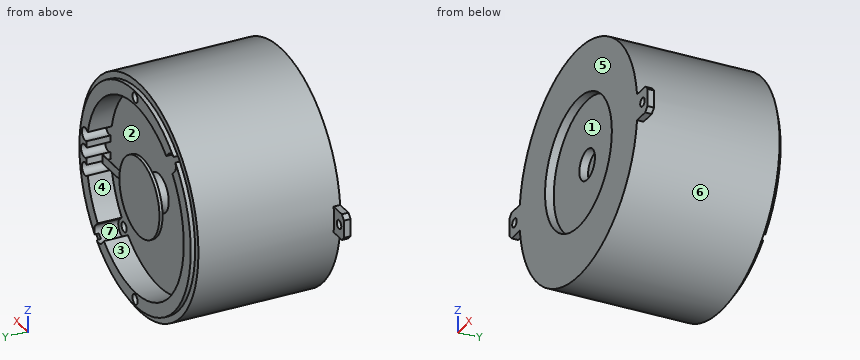
```python
from build123d import *

# Parameters (mm, degrees)
SKETCH_2_R              = 1
EXTRUDE_1_DEPTH         = 1.5
SKETCH_4_R              = 3.5
CUT_EXTRUDE_1_DEPTH     = 2
HOLE_WIZARD_M2_21_D     = 2.3
HOLE_WIZARD_M2_21_DEPTH = 10
HOLE_WIZARD_M2_21_TIP   = 0.690989712
HOLE_WIZARD_M2_22_D     = 2.3
HOLE_WIZARD_M2_22_DEPTH = 10
HOLE_WIZARD_M2_22_TIP   = 0.690989712
SKETCH_18_R             = 2
CUT_EXTRUDE_3_DEPTH     = 5.5
HOLE_WIZARD_M2_23_D     = 2.3
HOLE_WIZARD_M2_23_DEPTH = 15
HOLE_WIZARD_M2_23_TIP   = 0.690989712
CUT_EXTRUDE_START       = -5.5
SKETCH_20_R             = 1.5
CUT_EXTRUDE_4_DEPTH     = 5.5
SKETCH_8_W              = 2
SKETCH_8_H              = 0.05
EXTRUDE_3_DEPTH         = 18
SKETCH_9_R              = 2
CUT_EXTRUDE_2_DEPTH     = 5.5


# Read off the part's stored shape, not the designer's step: Повернуть1
with BuildPart() as part:
    # Повернуть1 outline → Повернуть1 (revolve)
    with BuildSketch(Plane.XY):
        Polygon((0, 26.1), (0, 0), (15, 0), (15, -2), (26.5, -2), (26.5, 30.6), (25, 30.6), (25, 31.6), (21.858230866, 31.6), (21.858230866, 26.1), align=None)
    revolve(axis=Axis((0, 0, 0), (0, 1, 0)))

    # Эскиз2 → Бобышка-Вытянуть1 (add)
    # profile 1 of 2: a face of its own
    with BuildSketch(Plane.XZ.offset(2)):
        Polygon((-31, -2), (-31, 2), (-30, 3), (-26.329641091, 3), (-26.329641091, -3), (-30, -3), align=None)
        with Locations(Location((-28.75, 0, 0), (0, 0, 270))):
            Circle(SKETCH_2_R, mode=Mode.SUBTRACT)
    # profile 2 of 2: a face of its own
    with BuildSketch(Plane.XZ.offset(2)):
        Polygon((30, 3), (26.329641091, 3), (26.329641091, -3), (30, -3), (31, -2), (31, 2), align=None)
        with Locations(Location((28.75, 0, 0), (0, 0, 90))):
            Circle(SKETCH_2_R, mode=Mode.SUBTRACT)
    extrude(amount=-EXTRUDE_1_DEPTH)

    # Эскиз4 → Вырез-Вытянуть1 (cut)
    with BuildSketch(Plane.XZ):
        with Locations(Location((0, 0, 0), (0, 0, 270))):
            Circle(SKETCH_4_R)
    extrude(amount=-CUT_EXTRUDE_1_DEPTH, mode=Mode.SUBTRACT)

    # Эскиз7 → Повернуть2 (revolve)
    with BuildSketch(Plane.XY, mode=Mode.PRIVATE) as revolve_2_sk:
        with BuildLine():
            Line((-1.963060758, 29.900525332), (-9, 29.900525332))
            Line((-9, 29.900525332), (-9, 30.6))
            Line((-9, 30.6), (0, 30.6))
            Line((0, 30.6), (0, 26.1))
            Line((0, 26.1), (-4.353608906, 26.1))
            add(Edge.make_bspline(
                [(-1.963060758, 29.900525332), (-2.24555005, 27.574534407), (-4.353608906, 26.1)],
                knots=[0, 0, 0, 1, 1, 1], degree=2))
        make_face()
    revolve(revolve_2_sk.sketch.rotate(Axis((0, 26.1, 0), (0, 1, 0)), 270), axis=Axis((0, 26.1, 0), (0, 1, 0)))

    # Сверло под метчик  спиральное M2.21
    with Locations(Plane(origin=(0, 31.6, 0), x_dir=(1, 0, 0), z_dir=(0, 1, 0))):
        with Locations((0, -23.523355069)):
            Hole(HOLE_WIZARD_M2_21_D / 2, depth=HOLE_WIZARD_M2_21_DEPTH)
            with Locations((0, 0, -(HOLE_WIZARD_M2_21_DEPTH + HOLE_WIZARD_M2_21_TIP / 2))):  # 118° drill point
                Cone(0, HOLE_WIZARD_M2_21_D / 2, HOLE_WIZARD_M2_21_TIP, mode=Mode.SUBTRACT)

    # Сверло под метчик  спиральное M2.22
    with Locations(Plane(origin=(0, 31.6, -23.5), x_dir=(0, 0, 1), z_dir=(0, 1, 0))):
        with Locations((0, 0)):
            Hole(HOLE_WIZARD_M2_22_D / 2, depth=HOLE_WIZARD_M2_22_DEPTH)
            with Locations((0, 0, -(HOLE_WIZARD_M2_22_DEPTH + HOLE_WIZARD_M2_22_TIP / 2))):  # 118° drill point
                Cone(0, HOLE_WIZARD_M2_22_D / 2, HOLE_WIZARD_M2_22_TIP, mode=Mode.SUBTRACT)

    # Эскиз18 → Вырез-Вытянуть3 (cut)
    with BuildSketch(Plane(origin=(0, 31.6, 0), x_dir=(1, 0, 0), z_dir=(0, 1, 0))):
        with Locations((15.708448043, 15.708448043)):
            Circle(SKETCH_18_R)
        with Locations((-15.708448043, -15.708448043)):
            Circle(SKETCH_18_R)
    extrude(amount=-CUT_EXTRUDE_3_DEPTH, mode=Mode.SUBTRACT)

    # Сверло под метчик  спиральное M2.23
    with Locations(Plane(origin=(-15.708448043, 31.6, 15.708448043), x_dir=(0, 0, 1), z_dir=(0, 1, 0))):
        with Locations((0, 0), (-31.416896086, 31.416896086)):
            Hole(HOLE_WIZARD_M2_23_D / 2, depth=HOLE_WIZARD_M2_23_DEPTH)
            with Locations((0, 0, -(HOLE_WIZARD_M2_23_DEPTH + HOLE_WIZARD_M2_23_TIP / 2))):  # 118° drill point
                Cone(0, HOLE_WIZARD_M2_23_D / 2, HOLE_WIZARD_M2_23_TIP, mode=Mode.SUBTRACT)

    # Эскиз20 → Вырез-Вытянуть4 (cut)
    with BuildSketch(Plane(origin=(0, 31.6, 0), x_dir=(1, 0, 0), z_dir=(0, 1, 0)).offset(CUT_EXTRUDE_START)):
        with Locations((22.760809842, 0)):
            Circle(SKETCH_20_R)
        with Locations((22.393028951, 4.075134238)):
            Circle(SKETCH_20_R)
        with Locations((22.393028951, -4.075134238)):
            Circle(SKETCH_20_R)
    extrude(amount=CUT_EXTRUDE_4_DEPTH, mode=Mode.SUBTRACT)

    # Эскиз8 → Бобышка-Вытянуть3 (add)
    with BuildSketch(Plane(origin=(0, 0, 0), x_dir=(0, 0, -1), z_dir=(1, 0, 0))):
        with Locations((0, 29.875525332)):
            Rectangle(SKETCH_8_W, SKETCH_8_H)
    extrude(amount=EXTRUDE_3_DEPTH)

    # Эскиз9 → Вырез-Вытянуть2 (cut)
    with BuildSketch(Plane(origin=(0, 31.6, 0), x_dir=(1, 0, 0), z_dir=(0, 1, 0)).offset(CUT_EXTRUDE_START)):
        with Locations((-16.330009516, -16.330009516)):
            Circle(SKETCH_9_R)
        with Locations((16.330009516, 16.330009516)):
            Circle(SKETCH_9_R)
    extrude(amount=CUT_EXTRUDE_2_DEPTH, mode=Mode.SUBTRACT)


solid = part.part
```
Build history of the part. All positions in model axes, mm. Face numbers are marked on the shaded views. A direction names the side the tool comes from. Coordinates: 2 decimals unless noted, no trailing zeros. Order: outer loops, then holes, each group sorted by start corner. A loop starts at its lowest first (then second) coordinate and runs counter-clockwise, first axis right, second up. Notation, with made-up numbers: (-11.75, 31) -> (25.25, 31) arc R15 cw to (25.25, 44) -> close; hole circle Ø5 at (12, 5.25). An arc over 180 degrees is marked (long way). Answer in a Markdown table with one row per item. Add a question column.
Q1. Which spindle directions (+Z, -Z, +X, -X, +Y, -Y) get a long thin tool onto all of the face, cutting with end or side? Do the marked faces 1, 2 and 3. Say none if no direction does.
Q2. Band-saw the part on C-C, the plane x = 7.5. List the corners of the cut face in (y, z), then the cut area to 3 significant figures.
Q3. Drop flat-ended pins along their axis: pin 1 (5 mm diameter, centred on x = -15, y = 6, fed in from -Z); pin 2 (3 mm diameter, centred on y = 17.5, z = 11, fed in from +X); pin 3 (3.5 mm diameter, centred on x = -28.5, z = -1.5, fed in from +Y). Give the stop position or say it passes through.
Q4. Wall check: line 1 along X through (y, z) = (-1.4, 0); line 2 along Z through (x, y) = (22.5, 29); line 3 along Y through (x, z) = (23.5, -10). Give the ranges that are in metal, low to high. Write a range as [from, to].
Q5. Band-saw the part on B-B, the plane y = 10. List the corners of the cut face in (x, z).
Q6. Mould opens along X. For the marked faces 4, 5, 6 and 7 say: +X half, -X half, draft (parallel to the pull), parting line (faces both ways), or undercut.
Q7. Band-saw the part on A-A, the plane x = -28.75. List the corners of the cut face in (y, z), then the cut area to 3 significant figures.
Q8. Band-saw the part on D-D, the plane y = 29. Give the number of separate pieces and of enclosed holes in the cut face, then the cut area to 3 significant figures.
Answers follow:
| question | item | result |
|---|---|---|
| 1 | face 1 | -Y |
| 1 | face 2 | none |
| 1 | face 3 | +Y |
| 2 | outline | (-2, -25.42) -> (30.6, -25.42) -> (30.6, -23.85) -> (31.6, -23.85) -> (31.6, -20.53) -> (26.1, -20.53) -> (26.1, 20.53) -> (31.6, 20.53) -> (31.6, 23.85) -> (30.6, 23.85) -> (30.6, 25.42) -> (-2, 25.42) -> (-2, 12.99) -> (0, 12.99) -> (0, -12.99) -> (-2, -12.99) -> close; (29.85, -1) -> (29.9, -1) -> (29.9, -4.97) -> (30.6, -4.97) -> (30.6, 4.97) -> (29.9, 4.97) -> (29.9, 1) -> (29.85, 1) -> close |
| 2 | area | 1,430 mm^2 |
| 3 | pin 1 | z = -23.37 |
| 3 | pin 2 | x = 24.74 |
| 3 | pin 3 | y = -0.5 |
| 4 | line 1 | [-31, -29.75], [-27.75, -15], [15, 27.75], [29.75, 31] |
| 4 | line 2 | [-14, -5.57], [-2.58, -1.48], [1.48, 2.58], [5.57, 14] |
| 4 | line 3 | [-2, 30.6] |
| 5 | outline | circle Ø53 at (0, 0) |
| 6 | face 4 | undercut |
| 6 | face 5 | draft |
| 6 | face 6 | parting line |
| 6 | face 7 | undercut |
| 7 | outline | (-2, -3) -> (-0.5, -3) -> (-0.5, -1) -> (-2, -1) -> close; (-2, 1) -> (-0.5, 1) -> (-0.5, 3) -> (-2, 3) -> close |
| 7 | area | 6.00 mm^2 |
| 8 | separate pieces | 2 |
| 8 | enclosed holes | 3 |
| 8 | area | 671 mm^2 |
